from build123d import *

# Parameters (mm, degrees)
CYLINDER076_R          = 1.6
CYLINDER076_DEPTH      = 6
CYLINDER076_ROLL_ANGLE = 90
CYLINDER074_R          = 1.25
CYLINDER074_DEPTH      = 6
CYLINDER074_ROLL_ANGLE = 90
BOX077_W               = 4.8
BOX077_H               = 2.8
BOX077_DEPTH           = 9.4
BOX075_W               = 237
BOX075_H               = 8
BOX075_DEPTH           = 15
BOX073_W               = 37
BOX073_H               = 160
BOX073_DEPTH           = 120
BOX073_PITCH_ANGLE     = -15
BOX068_W               = 475
BOX068_H               = 10
BOX068_DEPTH           = 10
BOX068_ROLL_ANGLE      = -27
BOX049_W               = 475
BOX049_H               = 8
BOX049_DEPTH           = 15
BOX069_W               = 475
BOX069_H               = 8
BOX069_DEPTH           = 15


with BuildPart() as cylinder076:
    # Cylinder076 → Cylinder076 (new body)
    with BuildSketch(Plane.XY):
        Circle(CYLINDER076_R)
    extrude(amount=CYLINDER076_DEPTH)


with BuildPart() as cylinder076_1:
    # Cylinder076 roll: moved
    add(cylinder076.part.rotate(Axis((0, 0, 0), (1, 0, 0)), CYLINDER076_ROLL_ANGLE))


with BuildPart() as cylinder076_2:
    # Cylinder076 placement: moved
    add(cylinder076_1.part.moved(Location((237.5, -40, 101))))


with BuildPart() as fusion087:
    # Cylinder074 → Cylinder074 (new body)
    with BuildSketch(Plane.XY):
        Circle(CYLINDER074_R)
    extrude(amount=CYLINDER074_DEPTH)


with BuildPart() as fusion087_1:
    # Cylinder074 roll: moved
    add(fusion087.part.rotate(Axis((0, 0, 0), (1, 0, 0)), CYLINDER074_ROLL_ANGLE))


with BuildPart() as fusion087_2:
    # Cylinder074 placement: moved
    add(fusion087_1.part.moved(Location((471, -40, 101))))

    # Fusion087: union Cylinder076
    add(cylinder076_2.part)


with BuildPart() as cube049:
    # Box077 → Box077 (new body)
    with BuildSketch(Plane(origin=(235.2, -42.8, 94.2), x_dir=(1, 0, 0), z_dir=(0, 0, 1))):
        with Locations((2.4, 1.4)):
            Rectangle(BOX077_W, BOX077_H)
    extrude(amount=BOX077_DEPTH)


with BuildPart() as cube047:
    # Box075 → Box075 (new body)
    with BuildSketch(Plane(origin=(3, -47, 90), x_dir=(1, 0, 0), z_dir=(0, 0, 1))):
        with Locations((118.5, 4)):
            Rectangle(BOX075_W, BOX075_H)
    extrude(amount=BOX075_DEPTH)


with BuildPart() as cube045:
    # Box073 → Box073 (new body)
    with BuildSketch(Plane.XY):
        with Locations((18.5, 80)):
            Rectangle(BOX073_W, BOX073_H)
    extrude(amount=BOX073_DEPTH)


with BuildPart() as cube045_1:
    # Box073 pitch: moved
    add(cube045.part.rotate(Axis((0, 0, 0), (0, 1, 0)), BOX073_PITCH_ANGLE))


with BuildPart() as cube045_2:
    # Box073 placement: moved
    add(cube045_1.part.moved(Location((502.2, -50, -4))))


with BuildPart() as cube040:
    # Box068 → Box068 (new body)
    with BuildSketch(Plane.XY):
        with Locations((237.5, 5)):
            Rectangle(BOX068_W, BOX068_H)
    extrude(amount=BOX068_DEPTH)


with BuildPart() as cube040_1:
    # Box068 roll: moved
    add(cube040.part.rotate(Axis((0, 0, 0), (1, 0, 0)), BOX068_ROLL_ANGLE))


with BuildPart() as cube040_2:
    # Box068 placement: moved
    add(cube040_1.part.moved(Location((0, -53.1, 85.5))))


with BuildPart() as cube021:
    # Box049 → Box049 (new body)
    with BuildSketch(Plane(origin=(0, -40, 89), x_dir=(1, 0, 0), z_dir=(0, 0, 1))):
        with Locations((237.5, 4)):
            Rectangle(BOX049_W, BOX049_H)
    extrude(amount=BOX049_DEPTH)


with BuildPart() as cut093:
    # Box069 → Box069 (new body)
    with BuildSketch(Plane(origin=(0, -47, 90), x_dir=(1, 0, 0), z_dir=(0, 0, 1))):
        with Locations((237.5, 4)):
            Rectangle(BOX069_W, BOX069_H)
    extrude(amount=BOX069_DEPTH)

    # Cut066: cut Cube021
    add(cube021.part, mode=Mode.SUBTRACT)

    # Cut067: cut Cube040
    add(cube040_2.part, mode=Mode.SUBTRACT)


with BuildPart() as cut093_1:
    # Cut067 placement: moved
    add(cut093.part.moved(Location((3, 0, 0))))

    # Cut080: cut Cube045
    add(cube045_2.part, mode=Mode.SUBTRACT)

    # Cut083: cut Cube047
    add(cube047.part, mode=Mode.SUBTRACT)

    # Fusion086: union Cube049
    add(cube049.part)

    # Cut093: cut Fusion087
    add(fusion087_2.part, mode=Mode.SUBTRACT)


solid = cut093_1.part
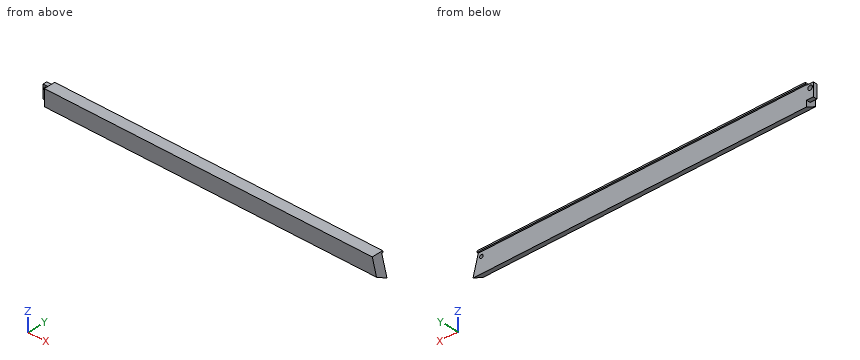
Input: part model. Units: mm. Frame: model coordinates. Give positions to 0.01 mm unless a question says otherwise; leave off trailing zeros. Order: outer loops, then holes, each group sorted by start corner. A loop starts at its lowest first (then second) coordinate and runs counter-clockwise, first axis right, second up. Notation, with made-up numbers: M 6.25,-39.5 L 50.25,-39.5 A21 cw 50.25,-0.5 Z; hole C 1,17 d10. An arc over 180 degrees is marked long. Answer as a JSON object with one key per item and string values.
1. Ray query, line 1 (X direction, y = -41.95, z = 101); line 2 (Z direction, x = 237.5, y = -41.4); line 3 (Y direction, x = 393, z = 96). Return the intervals inside material, ascending. Write a range as [from, to].
Result sheet:
{"line 1": "[235.2, 235.9], [239.1, 469.75], [472.25, 474.07]", "line 2": "[94.2, 99.4], [102.6, 103.6]", "line 3": "[-47, -40]"}
2. Cut plane A-A, the plane x = 278.5. Output: boundary loops of the cut face in (y, z), and give its area (3 significant figures).
Result sheet:
{"outline": "M -47,93.62 L -40,90.05 L -40,104 L -39,104 L -39,105 L -47,105 Z", "area": "93.2 mm²"}
3. First-contact query: P1, Ø1.1, axis at x = 341.5, y = -39.5, coming from the -Z side; P2, Ø3, axis at x = 471, z = 101, coming from the +Y side; P3, Ø1.5, axis at x = 347, y = -41, coming from the -Z side; P4, Ø3, axis at x = 237.5, z = 101, coming from the -Y side (3 decimals). Flat tips, straight axial feed; report the tip coordinate or a pass-through.
Result sheet:
{"P1": "z = 90.05", "P2": "y = -40", "P3": "z = 90.18", "P4": "through"}
4. Cut plane B-B, the plane y = -44.5. Output: boundary loops of the cut face in (x, z).
Result sheet:
{"outline": "M 240,92.34 L 476.39,92.34 L 472.99,105 L 240,105 Z; hole C 471,101 d2.5"}
